from build123d import *

# Parameters (mm, degrees)
CYLINDER018_R     = 2.6
CYLINDER018_DEPTH = 10
CYLINDER019_R     = 2.6
CYLINDER019_DEPTH = 10
CYLINDER017_R     = 2.6
CYLINDER017_DEPTH = 10
CYLINDER016_R     = 2.6
CYLINDER016_DEPTH = 10
BOX_W             = 120
BOX_H             = 120
BOX_DEPTH         = 3
SKETCH001_R       = 1.5
POCKET007_DEPTH   = 3.001


with BuildPart() as cilindro010:
    # Cylinder018 → Cylinder018 (new body)
    with BuildSketch(Plane(origin=(144.5, 152.1, 158), x_dir=(1, 0, 0), z_dir=(0, 0, 1))):
        Circle(CYLINDER018_R)
    extrude(amount=CYLINDER018_DEPTH)


with BuildPart() as cilindro011:
    # Cylinder019 → Cylinder019 (new body)
    with BuildSketch(Plane(origin=(79.5, 152.1, 158), x_dir=(1, 0, 0), z_dir=(0, 0, 1))):
        Circle(CYLINDER019_R)
    extrude(amount=CYLINDER019_DEPTH)


with BuildPart() as cilindro009:
    # Cylinder017 → Cylinder017 (new body)
    with BuildSketch(Plane(origin=(144.5, 114.1, 158), x_dir=(1, 0, 0), z_dir=(0, 0, 1))):
        Circle(CYLINDER017_R)
    extrude(amount=CYLINDER017_DEPTH)


with BuildPart() as cilindro008:
    # Cylinder016 → Cylinder016 (new body)
    with BuildSketch(Plane(origin=(79.5, 114.1, 158), x_dir=(1, 0, 0), z_dir=(0, 0, 1))):
        Circle(CYLINDER016_R)
    extrude(amount=CYLINDER016_DEPTH)


with BuildPart() as obj1:
    # Box → Box (new body)
    with BuildSketch(Plane(origin=(53, 45, 161), x_dir=(1, 0, 0), z_dir=(0, 0, 1))):
        with Locations((60, 60)):
            Rectangle(BOX_W, BOX_H)
    extrude(amount=BOX_DEPTH)

    # Cut008: cut Cilindro008
    add(cilindro008.part, mode=Mode.SUBTRACT)

    # Cut009: cut Cilindro009
    add(cilindro009.part, mode=Mode.SUBTRACT)

    # Cut010: cut Cilindro011
    add(cilindro011.part, mode=Mode.SUBTRACT)

    # Cut011: cut Cilindro010
    add(cilindro010.part, mode=Mode.SUBTRACT)

    # Sketch001 → Pocket007 (cut, through all)
    with BuildSketch(Plane.XY.offset(164)):
        with Locations((58, 50)):
            Circle(SKETCH001_R)
        with Locations((168, 50)):
            Circle(SKETCH001_R)
        with Locations((113, 150)):
            Circle(SKETCH001_R)
    extrude(amount=-POCKET007_DEPTH, mode=Mode.SUBTRACT)


solid = obj1.part
Read the model definition and answer for the solid it produces. Units are mm, in the model's axes. Round coordinates to 2 decimals unless told otherwise and drop trailing zeros. Write each loop counter-clockwise with the first axis right and the second up, starting at its lowest first coordinate (ties: lowest second). Pieces come first, ordered by that corner, then holes.
Q1. Find section C-C on x = 144.5. Determine the outline of the cut face in (y, z).
Values:
outline: (45, 161) - (111.5, 161) - (111.5, 164) - (45, 164) - close; (116.7, 161) - (149.5, 161) - (149.5, 164) - (116.7, 164) - close; (154.7, 161) - (165, 161) - (165, 164) - (154.7, 164) - close
Q2. Straight lines are drawn through the part: line 1 (X direction, y = 152.1, z = 161.85); line 2 (Y direction, x = 79.5, z = 162.55); line 3 (X direction, y = 154, z = 161.3). For each, find the intervals that lie inside material, in ascending order.
Values:
line 1: x = 53 to 76.9, 82.1 to 141.9, 147.1 to 173
line 2: y = 45 to 111.5, 116.7 to 149.5, 154.7 to 165
line 3: x = 53 to 77.73, 81.27 to 142.73, 146.27 to 173
Q3. Find section A-A on x = 113. Determine the outline of the cut face in (y, z).
Values:
outline: (45, 161) - (148.5, 161) - (148.5, 164) - (45, 164) - close; (151.5, 161) - (165, 161) - (165, 164) - (151.5, 164) - close
Q4. The mould has two halves that part along X. Classify faces 1 (the face through (53, 104, 162)), 2 (the face through (173, 104, 162)), 3 (the face through (146.98, 152.88, 162.48)), 4 (the face through (169.386, 49.425, 162.521)): released by +X, released by -X, zero draft, split by the parting line, or undercut.
Values:
face 1: released by -X
face 2: released by +X
face 3: undercut
face 4: undercut
Q5. A flat-ended cylindrical pin translates along its axis: P1, Ø2.5, axis at x = 168, y = 50, coming from the -Z side. Find the tip coordinate at first contact, or state that the pin passes through.
Values:
P1: passes through
Q6. Find section B-B on y = 50. Determine the outline of the cut face in (x, z), and give its area (3 significant figures).
Values:
outline: (53, 161) - (56.5, 161) - (56.5, 164) - (53, 164) - close; (59.5, 161) - (166.5, 161) - (166.5, 164) - (59.5, 164) - close; (169.5, 161) - (173, 161) - (173, 164) - (169.5, 164) - close
area: 342 mm2
